```python
from build123d import *

# Parameters (mm, degrees)
SKETCH1_W                       = 184
SKETCH1_H                       = 64
SKETCH1_W_2                     = 180
SKETCH1_H_2                     = 60
EXTRUDE_THIN1_DEPTH             = 30
SKETCH3_W                       = 184
SKETCH3_H                       = 64
BOSS_EXTRUDE1_DEPTH             = 2
SKETCH4_W                       = 174.419493498
SKETCH4_H                       = 4
CUT_EXTRUDE1_DEPTH              = 5
SKETCH5_W                       = 40.195784268
SKETCH5_H                       = 59.069599678
CUT_EXTRUDE2_DEPTH              = 15
SKETCH6_W                       = 44.195784268
SKETCH6_H                       = 67.776893145
SKETCH6_W_2                     = 40.195784268
SKETCH6_H_2                     = 63.776893145
EXTRUDE_THIN2_DEPTH             = 35
EXTRUDE_THIN2_DIRECTION_2_REACH = 118.55
SKETCH7_W                       = 128.018506196
SKETCH7_H                       = 58.604777903
CUT_EXTRUDE3_DEPTH              = 85
SKETCH8_W                       = 13
SKETCH8_H                       = 30
CUT_EXTRUDE4_DEPTH              = 85
SKETCH9_W                       = 44.195784268
SKETCH9_H                       = 65.776893145
BOSS_EXTRUDE2_DEPTH             = 2
SKETCH13_W                      = 20.06
SKETCH13_H                      = 40.06
CUT_EXTRUDE6_DEPTH              = 10
SKETCH18_R                      = 2.03
CUT_EXTRUDE8_DEPTH              = 10
SKETCH19_W                      = 50
SKETCH19_H                      = 40
CUT_EXTRUDE9_DEPTH              = 10
SKETCH20_R                      = 2.03
CUT_EXTRUDE10_DEPTH             = 10
SKETCH21_W                      = 37
SKETCH21_H                      = 32
CUT_EXTRUDE11_DEPTH             = 217


with BuildPart() as part:
    # Sketch1 → Extrude-Thin1 (new body)
    with BuildSketch(Plane(origin=(0, 0, 0), x_dir=(1, 0, 0), z_dir=(0, 1, 0))):
        Rectangle(SKETCH1_W, SKETCH1_H)
        Rectangle(SKETCH1_W_2, SKETCH1_H_2, mode=Mode.SUBTRACT)
    extrude(amount=EXTRUDE_THIN1_DEPTH)

    # Sketch3 → Boss-Extrude1 (add)
    with BuildSketch(Plane(origin=(0, 30, 0), x_dir=(1, 0, 0), z_dir=(0, 1, 0))):
        Rectangle(SKETCH3_W, SKETCH3_H)
    extrude(amount=BOSS_EXTRUDE1_DEPTH)

    # Sketch4 → Cut-Extrude1 (cut)
    with BuildSketch(Plane(origin=(0, 32, 0), x_dir=(1, 0, 0), z_dir=(0, 1, 0))):
        with Locations((0, -2)):
            Rectangle(SKETCH4_W, SKETCH4_H)
    extrude(amount=-CUT_EXTRUDE1_DEPTH, mode=Mode.SUBTRACT)

    # Sketch5 → Cut-Extrude2 (cut)
    with BuildSketch(Plane.XY.offset(32)):
        with Locations((0, 16)):
            Rectangle(SKETCH5_W, SKETCH5_H)
    extrude(amount=-CUT_EXTRUDE2_DEPTH, mode=Mode.SUBTRACT)

    # Sketch6 → Extrude-Thin2 (add)
    with BuildSketch(Plane.XY.offset(32)):
        with Locations((0, 31.888446573)):
            Rectangle(SKETCH6_W, SKETCH6_H)
        with Locations((0, 31.888446573)):
            Rectangle(SKETCH6_W_2, SKETCH6_H_2, mode=Mode.SUBTRACT)
    extrude(amount=EXTRUDE_THIN2_DEPTH)

    # Extrude-Thin2 direction 2: up to this face of the body (flat: up to its plane)
    extrude_thin2_direction_2_end = Plane(part.part.faces().sort_by_distance((0, 31, 17))[0])
    # Sketch6 → Extrude-Thin2 direction 2 (add, up to the picked face)
    with BuildSketch(Plane.XY.offset(32), mode=Mode.PRIVATE) as extrude_thin2_direction_2_sk1:
        with Locations((0, 31.888446573)):
            Rectangle(SKETCH6_W, SKETCH6_H)
        with Locations((0, 31.888446573)):
            Rectangle(SKETCH6_W_2, SKETCH6_H_2, mode=Mode.SUBTRACT)
    extrude_thin2_direction_2_tool1 = split(extrude(extrude_thin2_direction_2_sk1.sketch, amount=-EXTRUDE_THIN2_DIRECTION_2_REACH, mode=Mode.PRIVATE), bisect_by=extrude_thin2_direction_2_end, keep=Keep.BOTH, mode=Mode.PRIVATE)
    add(extrude_thin2_direction_2_tool1.solids().sort_by(Axis((0, -1.190866, 32), (0, 0, -1)))[0])

    # Sketch7 → Cut-Extrude3 (cut)
    with BuildSketch(Plane.XZ):
        with Locations((2.364457898, 44.353486129)):
            Rectangle(SKETCH7_W, SKETCH7_H)
    extrude(amount=CUT_EXTRUDE3_DEPTH, mode=Mode.SUBTRACT)

    # Sketch8 → Cut-Extrude4 (cut)
    with BuildSketch(Plane.ZY.offset(22.097892134)):
        with Locations((23.5, 15)):
            Rectangle(SKETCH8_W, SKETCH8_H)
    extrude(amount=-CUT_EXTRUDE4_DEPTH, mode=Mode.SUBTRACT)

    # Sketch9 → Boss-Extrude2 (add)
    with BuildSketch(Plane.XY.offset(67)):
        with Locations((0, 32.888446573)):
            Rectangle(SKETCH9_W, SKETCH9_H)
    extrude(amount=BOSS_EXTRUDE2_DEPTH)

    # Sketch13 → Cut-Extrude6 (cut)
    with BuildSketch(Plane.XY.offset(69)):
        with Locations((0, 30.776893145)):
            Rectangle(SKETCH13_W, SKETCH13_H)
    extrude(amount=-CUT_EXTRUDE6_DEPTH, mode=Mode.SUBTRACT)

    # Sketch18 → Cut-Extrude8 (cut)
    with BuildSketch(Plane.XY.offset(69)):
        with Locations((-5, 6.246893145)):
            Circle(SKETCH18_R)
        with Locations((5, 6.246893145)):
            Circle(SKETCH18_R)
    extrude(amount=-CUT_EXTRUDE8_DEPTH, mode=Mode.SUBTRACT)

    # Sketch19 → Cut-Extrude9 (cut)
    with BuildSketch(Plane.XY.offset(32)):
        with Locations((57.048946067, 0)):
            Rectangle(SKETCH19_W, SKETCH19_H)
    extrude(amount=-CUT_EXTRUDE9_DEPTH, mode=Mode.SUBTRACT)

    # Sketch20 → Cut-Extrude10 (cut)
    with BuildSketch(Plane.XY.offset(69)):
        with Locations((-5, 55.306893145)):
            Circle(SKETCH20_R)
        with Locations((5, 55.306893145)):
            Circle(SKETCH20_R)
    extrude(amount=-CUT_EXTRUDE10_DEPTH, mode=Mode.SUBTRACT)

    # Sketch21 → Cut-Extrude11 (cut)
    with BuildSketch(Plane.ZY.offset(22.097892134)):
        Polygon((72.732917278, 32), (69, 32), (69, 0), (32, 0), (32, -6.74330067), (76.348445097, -6.74330067), (76.348445097, 32), align=None)
        with Locations((50.5, 16)):
            Rectangle(SKETCH21_W, SKETCH21_H)
        Polygon((17, 65.776893145), (17, 32), (32, 32), (69, 32), (69, 65.776893145), align=None)
    extrude(amount=-CUT_EXTRUDE11_DEPTH, mode=Mode.SUBTRACT)


solid = part.part
```
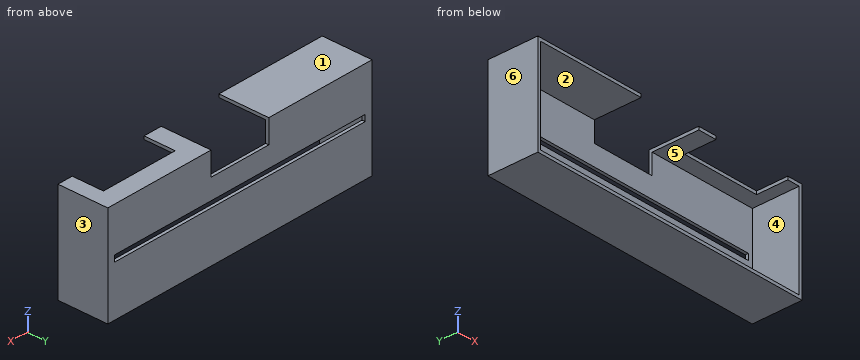
Can you work these out from the model? Positions are in its coordinate system, mm. Face numbers are marked on the shaded views. A direction names the side the tool comes from. Coordinates: 2 decimals unless noted, no trailing zeros. Loops run counter-clockwise (first coordinate to the right, second up) from the corner with the lowest first, then second, coordinate; pieces in that order, holes last.
Item 1: Suppose I cut it at D-D (z = -6.5). Please give me the cut outline in (x, y), then the cut area to 3 significant figures.
Answers below:
outline: (-92, 0) - (-90, 0) - (-90, 30) - (90, 30) - (90, 0) - (92, 0) - (92, 32) - (-92, 32) - close
area: 488 mm2
Item 2: If we mould it in two halves opening along X, with no side actions, what happens to the marked faces 3, 4, 5 and 6? For each: released by +X, released by -X, zero draft, split by the parting line, or undercut.
Answers below:
face 3: released by +X
face 4: undercut
face 5: undercut
face 6: released by -X
Item 3: Suppose I cut it at C-C (y = 9). Please give me the cut outline in (x, z), then the cut area to 3 significant figures.
Answers below:
outline: (-92, -32) - (92, -32) - (92, 32) - (82.05, 32) - (82.05, 30) - (90, 30) - (90, -30) - (-90, -30) - (-90, 30) - (-20.1, 30) - (-20.1, 32) - (-92, 32) - close; (20.1, 30) - (32.05, 30) - (32.05, 32) - (20.1, 32) - close
area: 796 mm2
Item 4: Suppose I cut it at A-A (x = 2). Please give me the cut outline in (y, z), then the cut area to 3 significant figures.
Answers below:
outline: (0, -32) - (32, -32) - (32, 0) - (30, 0) - (30, -30) - (0, -30) - close; (30, 4) - (32, 4) - (32, 17) - (30, 17) - close
area: 150 mm2
Item 5: I'm going to push flat-ended pins straight in: pin 1 (2 mm diameter, centred on x = -7, y = 31, fed in from +Z); pin 2 (1.5 mm diameter, centred on x = 17.5, y = 16, fed in from +Z); pin 3 (2 mm diameter, centred on x = 59, z = 31, fed in from -Y). Where does each tip first touch, or does it pass through?
Answers below:
pin 1: stops at z = 17
pin 2: stops at z = -30
pin 3: stops at y = 20
Item 6: Which directions (+Z, -Z, +X, -X, +Y, -Y) give clear straight access to the entire face, cutting with the end or side of a thin tool? Please do the marked faces 1 and 2.
Answers below:
face 1: +Z, +X, -X, +Y, -Y
face 2: -Y
Item 7: Suppose I cut it at B-B (z = 27.5). Please give me the cut outline in (x, y), then the cut area to 3 significant figures.
Answers below:
outline: (-92, 0) - (-90, 0) - (-90, 30) - (-20.1, 30) - (-20.1, 32) - (-92, 32) - close; (20.1, 30) - (90, 30) - (90, 0) - (92, 0) - (92, 32) - (20.1, 32) - close
area: 408 mm2
Item 8: Please list where these lines run through material, in increasing order: L1, parallel to X at y = 3.5, z = 29; L2, parallel to Z at x = -37, y = 31.5; L3, parallel to Z at x = 56.5, y = 22.
Answers below:
L1: x = -92 to -90, 90 to 92
L2: z = -32 to 0, 4 to 32
L3: z = -32 to -30, 30 to 32
